Geometry: final body of the model. Coordinates: model frame, mm. A direction names the side the tool comes from. Give positions to 0.01 mm unless a question says otherwise; leave off trailing zeros. Order: outer loops, then holes, each group sorted by start corner. A loop starts at its lowest first (then second) coordinate and runs counter-clockwise, first axis right, second up. Notation, with made-up numbers: (-0.75, 12) -> (39.25, 12) arc R24 ccw to (39.25, 33) -> close; hole circle Ø1 at (10, 39). An arc over 180 degrees is marked (long way). Write item = value, one per line.
```python
from build123d import *

# Parameters (mm, degrees)
F1_DEPTH = 152.4
F2_R     = 12.7
F3_DEPTH = 74.7069606938
F5_DEPTH = 76.2


with BuildPart() as f1:
    # F0 (on Right) → F1 (new body)
    with BuildSketch(Plane.YZ):
        Polygon((152.4, 50.8), (0, 50.8), (0, 0), (25.4, -35.4715141967), (152.4, 0), align=None)
    extrude(amount=F1_DEPTH)

    # F2 (on face) → F3 (cut, through all)
    with BuildSketch(Plane(origin=(0, 11.0284395164, -39.4855379111), x_dir=(1, 0, 0), z_dir=(0, 0.2690075997, -0.9631380541))):
        with Locations((101.6, -80.8519195663)):
            Circle(F2_R)
    extrude(amount=-F3_DEPTH, mode=Mode.SUBTRACT)

    # F4 (on face) → F5 (cut)
    with BuildSketch(Plane(origin=(0, 0, 0), x_dir=(0, -1, 0), z_dir=(-1, 0, 0))):
        Polygon((-152.4, 0), (-101.6, -14.1886056787), (-101.6, 34.35741062), (-152.4, 25.4), align=None)
    extrude(amount=-F5_DEPTH, mode=Mode.SUBTRACT)


solid = f1.part
```
1) Section query C-C (y = 105). Output: boundary loops of the cut face in (x, z).
Check sheet entries:
outline = (0, 33.76) -> (76.2, 33.76) -> (76.2, -13.24) -> (152.4, -13.24) -> (152.4, 50.8) -> (0, 50.8) -> close
2) First-contact query: P1, Ø2, axis at x = 56.5, z = -4, coming from the +Y side. Flat tip, straight axial feed; report the tip coordinate or a pass-through.
Check sheet entries:
P1 = 101.6
3) Reachability of faces 1 (the face through (38, 101.6, 10)), 2 (the face through (92, 152.4, 31)) from +Z, -Z, +X, -X, +Y, -Y: full face, straight path, thin tool, end or side. Return the list, or none.
Check sheet entries:
face_1 = -Z, -X
face_2 = +Z, -Z, +X, -X, +Y
4) Section query A-A (x = 65). Output: boundary loops of the cut face in (y, z).
Check sheet entries:
outline = (0, 0) -> (25.4, -35.47) -> (101.6, -14.19) -> (101.6, 34.36) -> (152.4, 25.4) -> (152.4, 50.8) -> (0, 50.8) -> close
5) Line query: line 1 (X direction, y = 110, z = -1.5); line 2 (X direction, y = 73.5, z = 22.5); line 3 (Y direction, x = 70, z = 5). Output: solid intervals per line, ascending. Write a range as from..to.
Check sheet entries:
line_1 = 76.2..152.4
line_2 = 0..89.55, 113.65..152.4
line_3 = 0..101.6
6) Section query B-B (x = 100.5). Output: boundary loops of the cut face in (y, z).
Check sheet entries:
outline = (0, 0) -> (25.4, -35.47) -> (76.71, -21.14) -> (56.62, 50.8) -> (0, 50.8) -> close; (82.89, 50.8) -> (101.09, -14.33) -> (152.4, 0) -> (152.4, 50.8) -> close
7) Mould query, pull axis Y, two halves, no side actions, for faces 3 (the face through (0, 58, 18)), 4 (the face through (99.947, 66.865, 14.349)), 5 (the face through (92.067, 73.9, -21.925)). Classes: +Y half, -Y half, draft (parallel to the pull), parting line (faces both ways), or undercut.
Check sheet entries:
face_3 = draft
face_4 = undercut
face_5 = +Y half
8) Section query D-D (x = 142). Output: boundary loops of the cut face in (y, z), plus the area to 3 significant figures.
Check sheet entries:
outline = (0, 0) -> (25.4, -35.47) -> (152.4, 0) -> (152.4, 50.8) -> (0, 50.8) -> close
area = 10,400 mm²
